Autodesk Inventor part; units mm, degrees
ref_plane "YZ Plane" through (0, 0, 0) normal (1, 0, 0) x (0, 1, 0)
ref_plane "XZ Plane" through (0, 0, 0) normal (0, 1, 0) x (-1, 0, 0)
ref_plane "XY Plane" through (0, 0, 0) normal (0, 0, 1) x (1, 0, 0)
sketch "Sketch1" plane through (0, 0, 0) normal (0, 0, 1) x (1, 0, 0)
  circle A0 centre (0, 0) radius 1.0795
  dimension "d0" = 2.159
extrude "Extrusion1" add sketch "Sketch1" along normal blind 10.16
sketch "Sketch2" plane through (0, 0, 0) normal (0, 0, -1) x (-1, 0, 0)
  circle A0 centre (0, 0) radius 2.54
  dimension "d3" = 5.08
extrude "Extrusion2" add sketch "Sketch2" along normal blind 1.905
fillet "Fillet1" radius 1.5875 1 edges at (2.54, 0, -1.905)
fillet "Fillet2" radius 0.3175 1 edges at (-1.0795, 0, 0)
fillet "Fillet3" radius 0.3175 1 edges at (2.54, 0, 0)
chamfer "Chamfer1" distance 0.3175 angle 45 1 edges at (-1.0795, 0, 10.16)
sketch "Sketch3" plane through (0, 0, -1.905) normal (0, 0, -1) x (-1, 0, 0)
  line L0 (-1.3748, 0) -> (-0.6874, 1.1906)
  line L1 (-0.6874, 1.1906) -> (0.6874, 1.1906)
  line L2 (0.6874, 1.1906) -> (1.3748, 0)
  line L3 (1.3748, 0) -> (0.6874, -1.1906)
  line L4 (0.6874, -1.1906) -> (-0.6874, -1.1906)
  line L5 (-0.6874, -1.1906) -> (-1.3748, 0)
  point P0 (0, 0)
  point P1 (0, 0)
  dimension "d17" = 2.3813
extrude "Extrusion3" cut sketch "Sketch3" against normal blind 0.635
thread "Thread1"
properties part number "Axel - Male" material "PPS Plastic"
Can you work these out from the model? Positions are in its coordinate system, mm. Give positions to 0.01 mm unless a question says otherwise; leave off trailing zeros. Loops run counter-clockwise (first coordinate to the right, second up) from the corner with the lowest first, then second, coordinate; pieces in that order, holes last. Notation, with made-up numbers: M 38,-1.5 L 92,-1.5 A26 cw 92,32.5 Z; hole C 62,8 d4. An arc over 180 degrees is marked long. One line per item, written item: value. Start each with the question number.
1) I'm going to push flat-ended pins straight in: pin 1 (2 mm diameter, centred on y = -1.5, z = 8.5, fed in from -X); pin 2 (3 mm diameter, centred on x = 0.5, z = 6.5, fed in from +Y); pin 3 (1.5 mm diameter, centred on x = -2, z = 4, fed in from +Y). Where does each tip first touch, or does it pass through?
2) Thinking about a two-plate mould opening in Y: for faces 1 (the face through (0, 0, -1.27)), 2 (the face through (-0.14, -1.07, 5.01)), 3 (the face through (0, 0, 10.16)), which applies, +Y half, -Y half, draft (parallel to the pull), parting line (faces both ways), or undercut?
3) If I drill on line 1 (Z direction, x = 0.5, y = -0.5); line 2 (Y direction, x = -0.1, z = 0.25); line 3 (Y direction, x = 0.35, z = -1), over which ranges is the centre line in solid material (lowest first)? Write a range as [from, to].
4) If we section it at A-A, the plane z = 8: Write out the boundary of the cut face in (x, y).
Completed:
1. pin 1: stops at x = -0.96
1. pin 2: stops at y = 1.08
1. pin 3: passes through
2. face 1: undercut
2. face 2: parting line
2. face 3: draft
3. line 1: z = [-1.27, 10.16]
3. line 2: y = [-1.08, 1.08]
3. line 3: y = [-2.36, 2.36]
4. outline: C 0,0 d2.16
